Design review of the part built by this model. Coordinates are the model's own, in mm. Face numbers are marked on the shaded views. A direction names the side the tool comes from. Round coordinates to 2 decimals unless told otherwise and drop trailing zeros. Write each loop counter-clockwise with the first axis right and the second up, starting at its lowest first coordinate (ties: lowest second). Pieces come first, ordered by that corner, then holes. Notation, with made-up numbers: M 15,44 L 56,44 A37 cw 56,80 Z; hole C 82,88.25 d8. An arc over 180 degrees is marked long. Use CSV: the item, a comma, the result in double quotes.
from build123d import *

# Parameters (mm, degrees)
SKETCH_1_W                    = 113.6
SKETCH_1_H                    = 166.2
EXTRUDE_1_DEPTH               = 1.6
EXTRUDE_2_DEPTH               = 69.5
SKETCH_3_W                    = 10
SKETCH_3_H                    = 163
EXTRUDE_3_DEPTH               = 6
SKETCH_20_R                   = 5
EXTRUDE_7_DEPTH               = 67.9
SKETCH_25_W                   = 9.6
SKETCH_25_H                   = 9.6
EXTRUDE_8_DEPTH               = 69.5
SKETCH_27_R                   = 1.55
CUT_EXTRUDE_1_DEPTH           = 6
EXTRUDE_9_DEPTH               = 1.6
SKETCH_30_R                   = 3.2
CUT_EXTRUDE_2_DEPTH           = 65.5
SKETCH_38_R                   = 1.7
CUT_EXTRUDE_9_DEPTH           = 3.9
SKETCH_31_R                   = 2.8
PATTERN_LINEAR_3_COUNT        = 2
PATTERN_LINEAR_3_PITCH        = 153.4
CUT_EXTRUDE_8_DEPTH           = 2
SKETCH_50_W                   = 0.9
SKETCH_50_H                   = 8.175007394
SKETCH_50_H_2                 = 1.824993516
SKETCH_50_H_3                 = 3.100006964
CUT_EXTRUDE_14_DEPTH          = 2
SKETCH_40_W                   = 5.2
SKETCH_40_H                   = 150.2
CUT_EXTRUDE_10_DEPTH          = 1.6
FILLET_2_R                    = 2
FILLET_3_R                    = 1
EXTRUDE_13_DEPTH              = 61.9
PATTERN_LINEAR_4_COUNT        = 2
PATTERN_LINEAR_4_PITCH        = 72
PATTERN_LINEAR_4_COPY_1_DEPTH = 61.9
SKETCH_17_R                   = 1.55
CUT_EXTRUDE_13_DEPTH          = 6
FILLET_4_R                    = 1


with BuildPart() as part:
    # Эскиз1 → Бобышка-Вытянуть1 (new body)
    with BuildSketch(Plane(origin=(0, 0, 0), x_dir=(1, 0, 0), z_dir=(0, 1, 0))):
        with Locations((-2.6, 0)):
            Rectangle(SKETCH_1_W, SKETCH_1_H)
    extrude(amount=-EXTRUDE_1_DEPTH)

    # Эскиз2 → Бобышка-Вытянуть2 (add)
    with BuildSketch(Plane(origin=(0, 0, 0), x_dir=(1, 0, 0), z_dir=(0, 1, 0))):
        Polygon((-54.2, 83.1), (54.2, 83.1), (54.2, -83.1), (-59.4, -83.1), (-59.4, -75.1), (-49.4, -75.1), (-49.4, -81.5), (52.6, -81.5), (52.6, 81.5), (-49.4, 81.5), (-49.4, 75.1), (-59.4, 75.1), (-59.4, 83.1), align=None)
    extrude(amount=EXTRUDE_2_DEPTH)

    # Эскиз3 → Бобышка-Вытянуть3 (add)
    with BuildSketch(Plane(origin=(0, 0, 0), x_dir=(1, 0, 0), z_dir=(0, 1, 0))):
        with Locations((27.6, 0)):
            Rectangle(SKETCH_3_W, SKETCH_3_H)
        with Locations((-44.4, 0)):
            Rectangle(SKETCH_3_W, SKETCH_3_H)
    extrude(amount=EXTRUDE_3_DEPTH)

    # Эскиз20 → Бобышка-Вытянуть7 (add)
    with BuildSketch(Plane(origin=(0, 0, 0), x_dir=(1, 0, 0), z_dir=(0, 1, 0))):
        with Locations(Location((-44.4, -66.5, 0), (0, 0, 180))):
            Circle(SKETCH_20_R)
        with Locations(Location((-44.390159066, 66.5, 0), (0, 0, 3.595357258))):
            Circle(SKETCH_20_R)
        with Locations(Location((27.6, 66.5, 0), (0, 0, 180))):
            Circle(SKETCH_20_R)
        with Locations(Location((27.6, -66.5, 0), (0, 0, 180))):
            Circle(SKETCH_20_R)
    extrude(amount=EXTRUDE_7_DEPTH)

    # Эскиз25 → Бобышка-Вытянуть8 (add)
    with BuildSketch(Plane(origin=(0, 0, 0), x_dir=(1, 0, 0), z_dir=(0, 1, 0))):
        with Locations((47.8, -76.7)):
            Rectangle(SKETCH_25_W, SKETCH_25_H)
        with Locations((47.8, 76.7)):
            Rectangle(SKETCH_25_W, SKETCH_25_H)
    extrude(amount=EXTRUDE_8_DEPTH)

    # Эскиз27 → Вырез-Вытянуть1 (cut)
    with BuildSketch(Plane(origin=(0, 67.9, 0), x_dir=(1, 0, 0), z_dir=(0, 1, 0))):
        with Locations(Location((-44.390159066, 66.5, 0), (0, 0, 270))):
            Circle(SKETCH_27_R)
        with Locations(Location((27.6, 66.5, 0), (0, 0, 270))):
            Circle(SKETCH_27_R)
        with Locations(Location((27.6, -66.5, 0), (0, 0, 270))):
            Circle(SKETCH_27_R)
        with Locations(Location((-44.4, -66.5, 0), (0, 0, 270))):
            Circle(SKETCH_27_R)
    extrude(amount=-CUT_EXTRUDE_1_DEPTH, mode=Mode.SUBTRACT)

    # Эскиз29 → Бобышка-Вытянуть9 (add)
    with BuildSketch(Plane(origin=(54.2, 0, 0), x_dir=(0, 0, -1), z_dir=(1, 0, 0))):
        with BuildLine():
            Line((35.331444881, 73.9), (54.368567283, 73.9))
            Line((54.368567283, 73.9), (54.458567283, 73.9))
            ThreePointArc((54.458567283, 73.9), (58.801220304, 75.698785778), (60.600006082, 80.041438799))
            Line((60.600006082, 80.041438799), (63.100006082, 80.041438799))
            Line((63.100006082, 80.041438799), (63.100006082, 69.5))
            Line((63.100006082, 69.5), (26.600006082, 69.5))
            Line((26.600006082, 69.5), (26.600006082, 80.041438799))
            Line((26.600006082, 80.041438799), (29.100006082, 80.041438799))
            ThreePointArc((29.100006082, 80.041438799), (30.89879186, 75.698785778), (35.241444881, 73.9))
            Line((35.241444881, 73.9), (35.331444881, 73.9))
        make_face()
    extrude(amount=-EXTRUDE_9_DEPTH)

    # Эскиз30 → Вырез-Вытянуть2 (cut)
    with BuildSketch(Plane.XZ.offset(1.6)):
        with Locations(Location((47.8, -76.7, 0), (0, 0, 270))):
            Circle(SKETCH_30_R)
    cut_extrude_2 = extrude(amount=-CUT_EXTRUDE_2_DEPTH, mode=Mode.SUBTRACT)

    # Эскиз38 → Вырез-Вытянуть9 (cut)
    with BuildSketch(Plane(origin=(0, 69.5, 0), x_dir=(1, 0, 0), z_dir=(0, 1, 0))):
        with Locations(Location((47.8, 76.7, 0), (0, 0, 270))):
            Circle(SKETCH_38_R)
    cut_extrude_9 = extrude(amount=-CUT_EXTRUDE_9_DEPTH, mode=Mode.SUBTRACT)

    # Эскиз31 → section 1 of loft_1
    with BuildSketch(Plane.XZ.offset(-63.9), mode=Mode.PRIVATE) as loft_1_s1:
        with Locations((47.8, -76.7)):
            Circle(SKETCH_31_R)
    # loft up to a face of the part (loft_1)
    loft_1 = loft([Face(Wire([part.edges().sort_by_distance((49.039246667, 65.6, -77.86373008))[0]])), loft_1_s1.sketch], mode=Mode.SUBTRACT)

    # Линейный массив3: Вырез-Вытянуть2, Вырез-Вытянуть9, Вырез-По сечениям1 ×2
    with Locations(*[(0, 0, i * PATTERN_LINEAR_3_PITCH) for i in range(1, PATTERN_LINEAR_3_COUNT)]):
        add(cut_extrude_2, mode=Mode.SUBTRACT)
        add(cut_extrude_9, mode=Mode.SUBTRACT)
        add(loft_1, mode=Mode.SUBTRACT)

    # Эскиз36 → Вырез-Вытянуть8 (cut)
    with BuildSketch(Plane(origin=(0, 69.5, 0), x_dir=(1, 0, 0), z_dir=(0, 1, 0))):
        Polygon((54.2, -82.4), (54.2, -83.1), (-54.2, -83.1), (-59.4, -83.1), (-59.4, -75.1), (-58.5, -75.1), (-58.5, -82.20017947), (-52.6, -82.20017947), (53.3, -82.20017947), (53.3, -67.20000355), (54.2, -67.20000355), align=None)
        Polygon((-54.2, 83.1), (54.2, 83.1), (54.2, 63.100006082), (53.3, 63.100006082), (53.3, 82.2), (-58.5, 82.2), (-58.5, 75.1), (-59.4, 75.1), (-59.4, 83.1), align=None)
    extrude(amount=-CUT_EXTRUDE_8_DEPTH, mode=Mode.SUBTRACT)

    # Эскиз50 → Вырез-Вытянуть14 (cut)
    with BuildSketch(Plane(origin=(0, 69.5, 0), x_dir=(1, 0, 0), z_dir=(0, 1, 0))):
        with Locations((53.05, 22.512502385)):
            Rectangle(SKETCH_50_W, SKETCH_50_H)
        with Locations((53.05, -34.18749901)):
            Rectangle(SKETCH_50_W, SKETCH_50_H_2)
        with Locations((53.05, -53.34999907)):
            Rectangle(SKETCH_50_W, SKETCH_50_H_3)
    extrude(amount=-CUT_EXTRUDE_14_DEPTH, mode=Mode.SUBTRACT)

    # Эскиз40 → Вырез-Вытянуть10 (cut)
    with BuildSketch(Plane(origin=(0, 0, 0), x_dir=(1, 0, 0), z_dir=(0, 1, 0))):
        with Locations((-56.8, 0)):
            Rectangle(SKETCH_40_W, SKETCH_40_H)
    extrude(amount=-CUT_EXTRUDE_10_DEPTH, mode=Mode.SUBTRACT)

    # Эскиз48 → Отверстие1 (revolve, cut)
    with BuildSketch(Plane(origin=(-53.9, 25, 83.1), x_dir=(0, -1, 0), z_dir=(1, 0, 0))):
        Polygon((0, 0), (0, 9), (1.55, 8.068666041), (1.55, 4.45), (3, 3), (3, 0), align=None)
    hole_wizard_1 = revolve(axis=Axis((-53.9, 25, 89.230023899), (0, 0, -1)), mode=Mode.SUBTRACT)

    # Зеркальное отражение5: Отверстие1 across plane
    add(hole_wizard_1.mirror(Plane.XY), mode=Mode.SUBTRACT)

    # Скругление2
    fillet_2_edges = [part.edges().sort_by_distance(p)[0] for p in [
        (43, 34.75, -71.9),
        (43, 34.75, 71.9),
    ]]
    fillet(fillet_2_edges, radius=FILLET_2_R)

    # Скругление3
    fillet_3_edges = [part.edges().sort_by_distance(p)[0] for p in [
        (54.2, 32.95, -83.1),
        (54.2, 32.95, 83.1),
        (-59.4, 32.95, 83.1),
        (-59.4, 32.95, -83.1),
    ]]
    fillet(fillet_3_edges, radius=FILLET_3_R)

    # Эскиз46 → Бобышка-Вытянуть13 (add)
    with BuildSketch(Plane(origin=(0, 6, 0), x_dir=(1, 0, 0), z_dir=(0, 1, 0))):
        Polygon((-45.4, 81.5), (-45.4, 71.396960413), (-43.4, 71.400977966), (-43.4, 81.5), align=None)
    extrude_13 = extrude(amount=EXTRUDE_13_DEPTH)

    # Зеркальное отражение4: Бобышка-Вытянуть13 across plane
    add(extrude_13.mirror(Plane.XY))

    # Линейный массив4: Бобышка-Вытянуть13 ×2
    with Locations(*[(i * PATTERN_LINEAR_4_PITCH, 0, 0) for i in range(1, PATTERN_LINEAR_4_COUNT)]):
        add(extrude_13)

    # Линейный массив4 copy 1 sketch → Линейный массив4 copy 1 (add)
    with BuildSketch(Plane(origin=(72, 6, 0), x_dir=(1, 0, 0), z_dir=(0, 1, 0))):
        Polygon((-45.4, -81.5), (-45.4, -71.396960413), (-43.4, -71.400977966), (-43.4, -81.5), align=None)
    extrude(amount=PATTERN_LINEAR_4_COPY_1_DEPTH)

    # Эскиз17 → Вырез-Вытянуть13 (cut)
    with BuildSketch(Plane(origin=(0, 6, 0), x_dir=(1, 0, 0), z_dir=(0, 1, 0))):
        with Locations(Location((27.1, 46.25, 0), (0, 0, 270))):
            Circle(SKETCH_17_R)
        with Locations(Location((-42.9, -46.25, 0), (0, 0, 270))):
            Circle(SKETCH_17_R)
    extrude(amount=-CUT_EXTRUDE_13_DEPTH, mode=Mode.SUBTRACT)

    # Скругление4
    fillet_4_edges = [part.edges().sort_by_distance(p)[0] for p in [
        (-59.4, -1.6, 78.6),
        (-2.6, -1.6, -83.1),
        (-59.4, -1.6, -78.6),
        (54.2, -1.6, 0),
        (-2.6, -1.6, 83.1),
        (-59.107106781, -1.6, 82.807106781),
        (53.907106781, -1.6, 82.807106781),
        (53.907106781, -1.6, -82.807106781),
        (-59.107106781, -1.6, -82.807106781),
    ]]
    fillet(fillet_4_edges, radius=FILLET_4_R)


solid = part.part
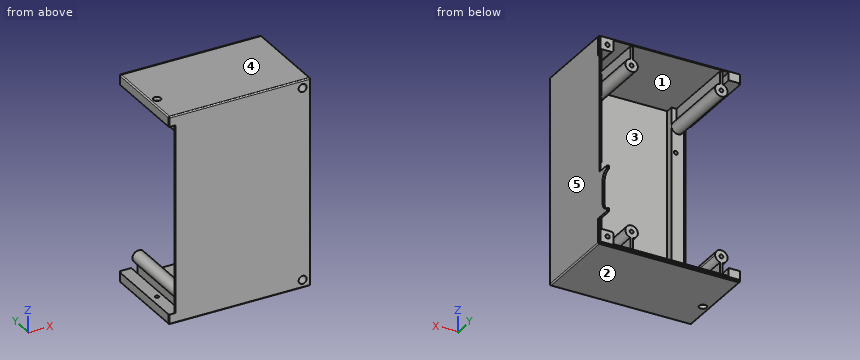
1) The part is to be moulded in two halves that separate along X. For the marked faces 3, 4 and 5, say which applies: released by +X, released by -X, zero draft, split by the parting line, or undercut.
Answers:
face 3,"undercut"
face 4,"zero draft"
face 5,"released by +X"
2) Add section A-A on x = 37.5. Write out the cut boundary in (y, z), then the cut area to 3 significant figures.
Answers:
outline,"M -1.6,-82.1 A1 ccw -0.6,-83.1 L 67.5,-83.1 L 67.5,-82.2 L 69.5,-82.2 L 69.5,-81.5 L 0,-81.5 L 0,81.5 L 69.5,81.5 L 69.5,82.2 L 67.5,82.2 L 67.5,83.1 L -0.6,83.1 A1 ccw -1.6,82.1 Z"
area,"484 mm²"
3) Add section C-C on y = 15. Give the number of separate pieces and of enclosed holes in the cut face, then the cut area to 3 significant figures.
Answers:
separate pieces,"1"
enclosed holes,"2"
area,"1,260 mm²"
4) Wall thickness on line 1 along X through (y, z) = (46.5, -76.7); line 2 along Z through (x, y) = (0.5, 4); line 3 along X through (y, z) = (2.5, 50.5): over which ranges is each line inside the solid? List them lowest first. Write a range as [from, to].
Answers:
line 1,"[-59.4, -49.4], [-45.4, -43.4], [26.6, 28.6], [43, 44.6], [51, 54.2]"
line 2,"[-83.1, -81.5], [81.5, 83.1]"
line 3,"[-49.4, -39.4], [22.6, 32.6], [52.6, 54.2]"
5) For pin 1 Ø1 at (x, y) = (4, 69.5) entering from +Z; pin 2 Ø1 at (x, z) = (40, 52.5) entering from +Y; pin 3 Ø1.3 at (x, y) = (53.5, 74.5) entering from -Z, all flat-tipped, find the tip position at first contact; note any pin that passes through.
Answers:
pin 1,"z = 82.2"
pin 2,"y = 0"
pin 3,"z = -63.1"
6) Add section B-B on z = 59. Write out the cut boundary in (x, y), then the cut area to 3 significant figures.
Answers:
outline,"M -54.2,-1.6 L 53.2,-1.6 A1 ccw 54.2,-0.6 L 54.2,69.5 L 52.6,69.5 L 52.6,0 L 32.6,0 L 32.6,6 L 22.6,6 L 22.6,0 L -39.4,0 L -39.4,6 L -49.4,6 L -49.4,0 L -54.2,0 Z"
area,"404 mm²"
7) Add section D-D on z = -50. Write out the cut boundary in (x, y).
Answers:
outline,"M -54.2,-1.6 L 53.2,-1.6 A1 ccw 54.2,-0.6 L 54.2,73.9 L 52.6,73.9 L 52.6,0 L 32.6,0 L 32.6,6 L 22.6,6 L 22.6,0 L -39.4,0 L -39.4,6 L -49.4,6 L -49.4,0 L -54.2,0 Z"
8) Machinability: for the marked faces 1 and 2, which of the approach directions +Z, -Z, +X, -X, +Y, -Y give a long, thin tool a straight path to every point of the face, cutting with its end or side? Answer none if there is none.
Answers:
face 1,"+Y"
face 2,"-Z, +X, -X, +Y, -Y"
